Can you work these out from the model? Positions are in its coordinate system, mm. Give positions to 0.01 mm unless a question says otherwise; leave off trailing zeros. Write each loop counter-clockwise with the first axis right and the second up, starting at its lowest first coordinate (ties: lowest second). Pieces come first, ordered by that corner, then holes.
```python
from build123d import *

# Parameters (mm, degrees)
BOSS_EXTRUDE1_DEPTH = 3
SKETCH2_W           = 3.2
SKETCH2_H           = 8.675
SKETCH2_H_2         = 8.875
SKETCH2_W_2         = 10.2
SKETCH2_H_3         = 3.2
CUT_EXTRUDE1_DEPTH  = 4


with BuildPart() as part:
    # Sketch1 → Boss-Extrude1 (new body)
    with BuildSketch(Plane(origin=(0, 0, 0), x_dir=(1, 0, 0), z_dir=(0, 1, 0))):
        Polygon((95.344434203, 0), (95.344434203, 25), (15, 25), (15, 0), (0, 0), (0, 52.05), (110.344434203, 52.05), (110.344434203, 0), align=None)
    extrude(amount=BOSS_EXTRUDE1_DEPTH)

    # Sketch2 → Cut-Extrude1 (cut, through all)
    with BuildSketch(Plane(origin=(0, 0, 0), x_dir=(1, 0, 0), z_dir=(0, 1, 0))):
        with Locations((1.5, 13.0125)):
            Rectangle(SKETCH2_W, SKETCH2_H)
        with Locations((1.5, 30.3625)):
            Rectangle(SKETCH2_W, SKETCH2_H)
        with Locations((1.5, 47.7125)):
            Rectangle(SKETCH2_W, SKETCH2_H_2)
        with Locations((35.172217102, 50.55)):
            Rectangle(SKETCH2_W_2, SKETCH2_H_3)
        with Locations((55.172217102, 31.5)):
            Rectangle(SKETCH2_W_2, SKETCH2_H_3)
        with Locations((55.172217102, 42.45)):
            Rectangle(SKETCH2_W_2, SKETCH2_H_3)
        with Locations((55.172217102, 50.55)):
            Rectangle(SKETCH2_W_2, SKETCH2_H_3)
        with Locations((15.172217102, 42.45)):
            Rectangle(SKETCH2_W_2, SKETCH2_H_3)
        with Locations((15.172217102, 50.55)):
            Rectangle(SKETCH2_W_2, SKETCH2_H_3)
        with Locations((35.172217102, 31.5)):
            Rectangle(SKETCH2_W_2, SKETCH2_H_3)
        with Locations((35.172217102, 42.45)):
            Rectangle(SKETCH2_W_2, SKETCH2_H_3)
        with Locations((108.844434203, 13.0125)):
            Rectangle(SKETCH2_W, SKETCH2_H)
        with Locations((95.172217102, 42.45)):
            Rectangle(SKETCH2_W_2, SKETCH2_H_3)
        with Locations((95.172217102, 50.55)):
            Rectangle(SKETCH2_W_2, SKETCH2_H_3)
        with Locations((108.844434203, 30.3625)):
            Rectangle(SKETCH2_W, SKETCH2_H)
        with Locations((75.172217102, 50.55)):
            Rectangle(SKETCH2_W_2, SKETCH2_H_3)
        with Locations((75.172217102, 42.45)):
            Rectangle(SKETCH2_W_2, SKETCH2_H_3)
        with Locations((75.172217102, 31.5)):
            Rectangle(SKETCH2_W_2, SKETCH2_H_3)
        with Locations((108.844434203, 50.55)):
            Rectangle(SKETCH2_W, SKETCH2_H_3)
    extrude(amount=CUT_EXTRUDE1_DEPTH, mode=Mode.SUBTRACT)


solid = part.part
```
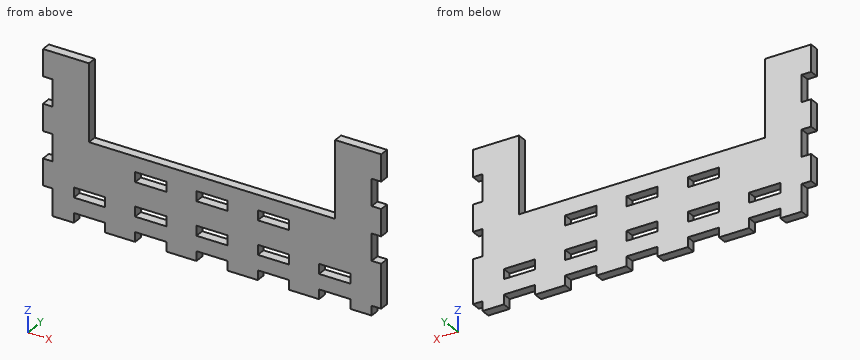
1) Please list where these lines run through material, in increasing order: L1, parallel to Z at x = 35, y = 1; L2, parallel to X at y = 2.25, z = -14; L3, parallel to X at y = 0.85, z = -41.
Values follow:
L1: z = -48.95 to -44.05, -40.85 to -33.1, -29.9 to -25
L2: x = 3.1 to 15, 95.34 to 107.24
L3: x = 0 to 10.07, 20.27 to 30.07, 40.27 to 50.07, 60.27 to 70.07, 80.27 to 90.07, 100.27 to 110.34
2) Suppose I cut it at C-C on x = 13. Write out the boundary of the cut face in (y, z).
Values follow:
outline: (0, -48.95) - (3, -48.95) - (3, -44.05) - (0, -44.05) - close; (0, -40.85) - (3, -40.85) - (3, 0) - (0, 0) - close
3) Suppose I cut it at A-A on x = 73.5. Write out the boundary of the cut face in (y, z).
Values follow:
outline: (0, -48.95) - (3, -48.95) - (3, -44.05) - (0, -44.05) - close; (0, -40.85) - (3, -40.85) - (3, -33.1) - (0, -33.1) - close; (0, -29.9) - (3, -29.9) - (3, -25) - (0, -25) - close
4) Suppose I cut it at D-D on y = 0.8. State how many separate pieces and enclosed holes the cut face has, plus the area to 3 significant figures.
Values follow:
separate pieces: 1
enclosed holes: 8
area: 3,170 mm2
5) Suppose I cut it at B-B on z = -13.5. Write out the boundary of the cut face in (x, y), plus the area to 3 significant figures.
Values follow:
outline: (3.1, 0) - (15, 0) - (15, 3) - (3.1, 3) - close; (95.34, 0) - (107.24, 0) - (107.24, 3) - (95.34, 3) - close
area: 71.4 mm2
6) For pin 1 Ø0.9 at (y, z) = (2, -31.5) entering from -X; pin 2 Ø1.5 at (x, y) = (12.5, 2) entering from -Z; pin 3 Ø1.5 at (y, z) = (1, -31) entering from +X, each with a flat end and sliding along its axis, tell me the tip position at first contact or that it passes through.
Values follow:
pin 1: stops at x = 3.1
pin 2: stops at z = -48.95
pin 3: stops at x = 107.24
